Part model, mm, in its own coordinate system. A direction names the side the tool comes from. Give positions to 0.01 mm unless a question says otherwise; leave off trailing zeros. Write each loop counter-clockwise with the first axis right and the second up, starting at its lowest first coordinate (ties: lowest second). Pieces come first, ordered by that corner, then holes. Notation, with made-up numbers: (-1, -21.5) - (29, -21.5) arc R17 cw to (29, 5.5) - close; hole circle Ø4 at (-5, 81.25). An arc over 180 degrees is marked (long way). Answer in a Markdown table with one row per item. Add a question column.
1. Band-saw the part on C-C on z = 0.25. Write the cut outline in (x, y) (3 decimals), plus the area to 3 significant figures.
2. Band-saw the part on A-A on z = 1.2. Write the cut outline in (x, y) (3 decimals), plus the area to 3 significant figures.
3. Which spindle directions (+Z, -Z, +X, -X, +Y, -Y) get a long thin tool onto all of the face, cutting with end or side? Do faces 1 (the flat face through (0, 2, 2.032)), 2 (the flat face through (-1, 3, 0)). Say none if no direction does.
4. Band-saw the part on B-B on x = 0. Write the cut outline in (y, z).
5. Probe line 1 along Y through (x, z) = (0, 1.35); line 2 along Z through (x, y) = (0.2, 2.5); line 3 along X through (y, z) = (0.25, 1.25). List the from-to ranges inside material, lowest first.
6. Drop flat-ended pins along their axis: pin 1 Ø1.5 at (x, z) = (-2, 1) entering from -Y; pin 2 Ø1.6 at (x, y) = (0, 0) entering from -Z; pin 3 Ø1.2 at (x, y) = (0, 2) entering from +Z. Give the stop position or say it passes through.
7. Pull direction Y, two halves, no side cores. Call faces 3 (the flat face through (0, 2, 0.508)), 4 (the flat face through (-1, 3, 2.54)), 5 (the cylindrical face through (-1.967, 5.68, 1.252)): released by +Y, released by -Y, zero draft, split by the parting line, or undercut.
```python
from build123d import *

# Parameters (mm, degrees)
SKETCH2_R           = 1.016
BOSS_EXTRUDE2_DEPTH = 2.54
CUT_EXTRUDE1_DEPTH  = 0.508
CUT_EXTRUDE2_DEPTH  = 0.508


with BuildPart() as part:
    # Sketch2 → Boss-Extrude2 (new body)
    with BuildSketch(Plane.XY):
        with BuildLine():
            ThreePointArc((-2.54, 0), (0, -2.54), (2.54, 0))
            Line((2.54, 0), (2.54, 4.318))
            ThreePointArc((2.54, 4.318), (1.982038418, 5.665038418), (0.635, 6.223))
            Line((0.635, 6.223), (-0.635, 6.223))
            ThreePointArc((-0.635, 6.223), (-1.982038418, 5.665038418), (-2.54, 4.318))
            Line((-2.54, 4.318), (-2.54, 0))
        make_face()
        Circle(SKETCH2_R, mode=Mode.SUBTRACT)
    extrude(amount=BOSS_EXTRUDE2_DEPTH)

    # Sketch3 → Cut-Extrude1 (cut)
    with BuildSketch(Plane.XY.offset(2.54)):
        with BuildLine():
            Line((-0.762, 2.423005572), (-0.762, 1.319822715))
            ThreePointArc((-0.762, 1.319822715), (0, 1.524), (0.762, 1.319822715))
            Line((0.762, 1.319822715), (0.762, 2.423005572))
            ThreePointArc((0.762, 2.423005572), (0, 2.54), (-0.762, 2.423005572))
        make_face()
        with BuildLine():
            Line((-0.762, 3.556), (-0.762, 2.423005572))
            ThreePointArc((-0.762, 2.423005572), (0, 2.54), (0.762, 2.423005572))
            Line((0.762, 2.423005572), (0.762, 3.556))
            Line((0.762, 3.556), (-0.762, 3.556))
        make_face()
        with BuildLine():
            Line((-0.762, 1.319822715), (-0.762, 0.672020833))
            ThreePointArc((-0.762, 0.672020833), (0, 1.016), (0.762, 0.672020833))
            Line((0.762, 0.672020833), (0.762, 1.319822715))
            ThreePointArc((0.762, 1.319822715), (0, 1.524), (-0.762, 1.319822715))
        make_face()
    extrude(amount=-CUT_EXTRUDE1_DEPTH, mode=Mode.SUBTRACT)

    # Sketch4 → Cut-Extrude2 (cut)
    with BuildSketch(Plane(origin=(0, 0, 0), x_dir=(-1, 0, 0), z_dir=(0, 0, -1))):
        with BuildLine():
            ThreePointArc((-0.762, 2.423005572), (0, 2.54), (0.762, 2.423005572))
            Line((0.762, 2.423005572), (0.762, 3.556))
            Line((0.762, 3.556), (-0.762, 3.556))
            Line((-0.762, 3.556), (-0.762, 2.423005572))
        make_face()
        with BuildLine():
            Line((0.762, 1.319822715), (0.762, 2.423005572))
            ThreePointArc((0.762, 2.423005572), (0, 2.54), (-0.762, 2.423005572))
            Line((-0.762, 2.423005572), (-0.762, 1.319822715))
            ThreePointArc((-0.762, 1.319822715), (0, 1.524), (0.762, 1.319822715))
        make_face()
        with BuildLine():
            Line((0.762, 0.672020833), (0.762, 1.319822715))
            ThreePointArc((0.762, 1.319822715), (0, 1.524), (-0.762, 1.319822715))
            Line((-0.762, 1.319822715), (-0.762, 0.672020833))
            ThreePointArc((-0.762, 0.672020833), (0, 1.016), (0.762, 0.672020833))
        make_face()
    extrude(amount=-CUT_EXTRUDE2_DEPTH, mode=Mode.SUBTRACT)

    # Sketch7 → Cut-Revolve1 (revolve, cut)
    with BuildSketch(Plane(origin=(0, 0, 0), x_dir=(1, 0, 0), z_dir=(0, 1, 0))):
        Polygon((0, 0), (0, -2.54), (1.524, -2.54), (0.508, -1.524), (0.508, -1.016), (1.524, 0), align=None)
    revolve(axis=Axis((0, 0, 0), (0, 0, 1)), mode=Mode.SUBTRACT)


solid = part.part
```
Values:
| question | item | result |
|---|---|---|
| 1 | outline | (-2.54, 0) arc R2.54 ccw to (2.54, 0) - (2.54, 4.318) arc R1.905 ccw to (0.635, 6.223) - (-0.635, 6.223) arc R1.905 ccw to (-2.54, 4.318) - close; hole (-0.762, 1.021) arc R1.274 ccw (long way) to (0.762, 1.021) - (0.762, 3.556) - (-0.762, 3.556) - close |
| 1 | area | 31.5 mm² |
| 2 | outline | (-2.54, 0) arc R2.54 ccw to (2.54, 0) - (2.54, 4.318) arc R1.905 ccw to (0.635, 6.223) - (-0.635, 6.223) arc R1.905 ccw to (-2.54, 4.318) - close; hole circle Ø2.032 at (0, 0) |
| 2 | area | 36.9 mm² |
| 3 | face 1 | +Z |
| 3 | face 2 | -Z, +X, -X, +Y, -Y |
| 4 | outline | (-2.54, 0) - (-1.52, 0) - (-1.02, 0.51) - (-1.02, 2.03) - (-1.52, 2.54) - (-2.54, 2.54) - close; (1.02, 0.51) - (3.56, 0.51) - (3.56, 0) - (6.22, 0) - (6.22, 2.54) - (3.56, 2.54) - (3.56, 2.03) - (1.02, 2.03) - close |
| 5 | line 1 | y = -2.54 to -1.02, 1.02 to 6.22 |
| 5 | line 2 | z = 0.51 to 2.03 |
| 5 | line 3 | x = -2.54 to -0.98, 0.98 to 2.54 |
| 6 | pin 1 | stops at y = -2.21 |
| 6 | pin 2 | passes through |
| 6 | pin 3 | stops at z = 2.03 |
| 7 | face 3 | undercut |
| 7 | face 4 | zero draft |
| 7 | face 5 | released by +Y |
